from build123d import *

# Parameters (mm, degrees)
CROQUIS1_W              = 50.8
CROQUIS1_H              = 85
SALIENTE_EXTRUIR1_DEPTH = 9.525
CROQUIS2_R              = 13
CORTAR_EXTRUIR1_DEPTH   = 51.419595645
CROQUIS3_R              = 1.55
CROQUIS3_R_2            = 1.6
CORTAR_EXTRUIR2_DEPTH   = 51.419595645
CROQUIS4_R              = 2
CORTAR_EXTRUIR3_DEPTH   = 51.419595645
CROQUIS5_W              = 50.8
CROQUIS5_H              = 12.7
CORTAR_EXTRUIR4_DEPTH   = 51.419595645
CROQUIS6_W              = 50.8
CROQUIS6_H              = 9.525
SALIENTE_EXTRUIR2_DEPTH = 84.8


with BuildPart() as part:
    # Croquis1 → Saliente-Extruir1 (new body)
    with BuildSketch(Plane(origin=(0, 0, 0), x_dir=(1, 0, 0), z_dir=(0, 1, 0))):
        Rectangle(CROQUIS1_W, CROQUIS1_H)
    extrude(amount=SALIENTE_EXTRUIR1_DEPTH)

    # Croquis2 → Cortar-Extruir1 (cut, through all)
    with BuildSketch(Plane.XZ):
        with Locations(Location((0, -21.35, 0), (0, 0, 270))):
            Circle(CROQUIS2_R)
    extrude(amount=-CORTAR_EXTRUIR1_DEPTH, mode=Mode.SUBTRACT)

    # Croquis3 → Cortar-Extruir2 (cut, through all)
    with BuildSketch(Plane.XZ):
        with Locations(Location((-15.5, -5.85, 0), (0, 0, 270))):
            Circle(CROQUIS3_R)
        with Locations(Location((15.5, -5.85, 0), (0, 0, 270))):
            Circle(CROQUIS3_R)
        with Locations(Location((15.5, -36.85, 0), (0, 0, 270))):
            Circle(CROQUIS3_R)
        with Locations(Location((-15.5, -36.85, 0), (0, 0, 270))):
            Circle(CROQUIS3_R_2)
    extrude(amount=-CORTAR_EXTRUIR2_DEPTH, mode=Mode.SUBTRACT)

    # Croquis4 → Cortar-Extruir3 (cut, through all)
    with BuildSketch(Plane(origin=(0, 9.525, 0), x_dir=(1, 0, 0), z_dir=(0, 1, 0))):
        with Locations(Location((-19, 21.35, 0), (0, 0, 270))):
            Circle(CROQUIS4_R)
        with Locations(Location((19, 21.35, 0), (0, 0, 270))):
            Circle(CROQUIS4_R)
        with Locations(Location((0, 2.35, 0), (0, 0, 270))):
            Circle(CROQUIS4_R)
    extrude(amount=-CORTAR_EXTRUIR3_DEPTH, mode=Mode.SUBTRACT)

    # Croquis5 → Cortar-Extruir4 (cut, through all)
    with BuildSketch(Plane(origin=(0, 9.525, 0), x_dir=(1, 0, 0), z_dir=(0, 1, 0))):
        with Locations((0, -36.15)):
            Rectangle(CROQUIS5_W, CROQUIS5_H)
    extrude(amount=-CORTAR_EXTRUIR4_DEPTH, mode=Mode.SUBTRACT)

    # Croquis6 → Saliente-Extruir2 (add)
    with BuildSketch(Plane(origin=(0, 9.525, 0), x_dir=(1, 0, 0), z_dir=(0, 1, 0))):
        with Locations((0, -25.0375)):
            Rectangle(CROQUIS6_W, CROQUIS6_H)
    extrude(amount=SALIENTE_EXTRUIR2_DEPTH)


solid = part.part
Check sheet for the modelled part. Datum: model origin and axes. Units: mm. A direction names the side the tool comes from. Round coordinates to 2 decimals unless told otherwise and drop trailing zeros. Order: outer loops, then holes, each group sorted by start corner. A loop starts at its lowest first (then second) coordinate and runs counter-clockwise, first axis right, second up. Notation, with made-up numbers: M -40,77.25 L -12,77.25 A25 ccw -12,104.25 Z; hole C 84,56.25 d2. An arc over 180 degrees is marked long. One line per item, written item: value. Start each with the question number.
1. Section check C-C on x = 4.5. Enter the section's corners in (y, z) (3 decimals).
2. Section check B-B on x = 19. Enter the section's corners in (y, z) (3 decimals).
3. Release check for a two-part mould opening along X. For faces 3 (the flat face through (-25.4, 33, 21)), 4 (the cylindrical face through (-0.766, 4.829, -0.503)), 5 (the flat face through (0, 5, -42.5)), 6 (the cylindrical face through (20.7, 4.8, -20.3)) record: released by +X, released by -X, zero draft, split by the parting line, or undercut.
4. Gauge pin test, flat ends, axial feed: P1, Ø8, axis at x = -7.5, z = -21, coming from the +Y side; P2, Ø12, axis at x = 17, y = 75, coming from the -Z side (3 decimals); P3, Ø5, axis at x = 19, z = -21.35, coming from the +Y side (3 decimals). Record the tip position at first contact, or that the pin passes through.
5. Access from +Z, -Z, +X, -X, +Y, -Y to the whole of each face (thin tool, end or side, straight path). Record for faces 1 (the flat face through (0, 0, -7)), 2 (the flat face through (0, 9.525, -5)).
6. Section check D-D on z = -33. Enter the section's corners in (x, y) (3 decimals).
7. Section check A-A on z = -2.35. Enter the section's corners in (x, y) (3 decimals).
8. Scan lines: line 1 along X through (y, z) = (7.75, -21.35); line 2 along X through (y, z) = (5, -36.85); line 3 along Z through (x, y) = (15, 7). Record each from-to range of solid material in increasing order.
Results found:
1. outline: M 0,-42.5 L 9.525,-42.5 L 9.525,-33.546 L 0,-33.546 Z; M 0,-9.154 L 9.525,-9.154 L 9.525,20.275 L 94.325,20.275 L 94.325,29.8 L 0,29.8 Z
2. outline: M 0,-42.5 L 9.525,-42.5 L 9.525,-23.35 L 0,-23.35 Z; M 0,-19.35 L 9.525,-19.35 L 9.525,20.275 L 94.325,20.275 L 94.325,29.8 L 0,29.8 Z
3. face 3: released by -X
3. face 4: undercut
3. face 5: zero draft
3. face 6: undercut
4. P1: through
4. P2: z = 20.275
4. P3: y = 9.525
5. face 1: +Z, -Z, +X, -X, -Y
5. face 2: -Z, +X, -X, +Y
6. outline: M -25.4,0 L -5.769,0 L -5.769,9.525 L -25.4,9.525 Z; M 5.769,0 L 25.4,0 L 25.4,9.525 L 5.769,9.525 Z
7. outline: M -25.4,0 L -2,0 L -2,9.525 L -25.4,9.525 Z; M 2,0 L 25.4,0 L 25.4,9.525 L 2,9.525 Z
8. line 1: -25.4 to -21, -17 to -13, 13 to 17, 21 to 25.4
8. line 2: -25.4 to -17.1, -13.9 to 13.95, 17.05 to 25.4
8. line 3: -42.5 to -38.32, -35.38 to -7.32, -4.38 to 29.8
